CAD build for the part. Positions are in the model's coordinates, mm. Face numbers are marked on the shaded views. A direction names the side the tool comes from. Round coordinates to 2 decimals unless told otherwise and drop trailing zeros. Write each loop counter-clockwise with the first axis right and the second up, starting at its lowest first coordinate (ties: lowest second). Pieces come first, ordered by that corner, then holes. Notation, with made-up numbers: (26.5, 82) -> (67.5, 82) arc R28 ccw to (67.5, 121) -> close; hole circle Ø10 at (51.25, 38.5). An arc over 180 degrees is marked (long way). Put each result on its own line as item: value. Start each with the question number.
1. Saw through at D-D on x = 56.5. List the corners of the cut face in (y, z), and give its area (3 significant figures).
2. Saw through at A-A on y = 4.5. List the corners of the cut face in (x, z).
3. Saw through at B-B on z = 2.25. List the corners of the cut face in (x, y).
4. Saw through at C-C on x = 12.5. List the corners of the cut face in (y, z), and give its area (3 significant figures).
5. Pull direction X, two halves, no side cores. Call the marked faces 3, 4 and 5: pulls with the +X half, pulls with the -X half, needs draft (parallel to the pull), parting line crosses it, or undercut.
6. Flat gauge pins, fed straight in: P1, Ø1.2, axis at x = 2, z = 0.5, coming from the +Y side; P2, Ø3, axis at y = 0.5, z = 2.5, coming from the +X side; P3, Ø4, axis at y = 6, z = -3.5, coming from the +X side; P4, Ø4, axis at y = 6, z = 6, coming from the +X side. Where does each tip first touch, or does it go through?
7. Drill centre lines: line 1 (X direction, y = 0.25, z = 4.75); line 2 (Y direction, x = 49, z = 1.5); line 3 (X direction, y = 2, z = -5.25). Where is each one in solid material? Low to high. Write a range as from..to.
8. 3-axis set-ups, long thin cutter, end or side, ignore diameter. For the marked faces 1 and 2: which of +Z, -Z, +X, -X, +Y, -Y reach the whole face in a straight line?
from build123d import *

# Parameters (mm, degrees)
BOSS_EXTRUDE1_DEPTH = 5.5
SKETCH2_W           = 53.34
SKETCH2_H           = 3
BOSS_EXTRUDE2_DEPTH = 13.95
SCALE1_SCALE        = 0.98


with BuildPart() as part:
    # Sketch1 → Boss-Extrude1 (new, symmetric)
    with BuildSketch(Plane.XY):
        with BuildLine():
            Line((0, 0), (2.5, 0))
            Line((2.5, 0), (2.5, -0.54))
            Line((2.5, -0.54), (55.84, -0.54))
            Line((55.84, -0.54), (55.84, 1.698))
            Line((55.84, 1.698), (57.84, 1.698))
            Line((57.84, 1.698), (58.54, 1.698))
            ThreePointArc((58.54, 1.698), (59.247106781, 1.990893219), (59.54, 2.698))
            Line((59.54, 2.698), (59.54, 7.579046555))
            ThreePointArc((59.54, 7.579046555), (61.34, 9.379046555), (63.14, 7.579046555))
            Line((63.14, 7.579046555), (63.14, -0.54))
            Line((63.14, -0.54), (66.14, -0.54))
            Line((66.14, -0.54), (66.14, 0.46))
            Line((66.14, 0.46), (63.84, 0.46))
            Line((63.84, 0.46), (63.84, 2.16))
            Line((63.84, 2.16), (65.34, 2.16))
            Line((65.34, 2.16), (63.84, 7.758076211))
            Line((63.84, 7.758076211), (63.84, 7.579046555))
            ThreePointArc((63.84, 7.579046555), (61.34, 10.079046555), (58.84, 7.579046555))
            Line((58.84, 7.579046555), (58.84, 2.46))
            Line((58.84, 2.46), (55.84, 2.46))
            Line((55.84, 2.46), (2.5, 2.46))
            Line((2.5, 2.46), (2.5, 0.5))
            Line((2.5, 0.5), (0, 0.5))
            Line((0, 0.5), (0, 0))
        make_face()
    extrude(amount=BOSS_EXTRUDE1_DEPTH, both=True)

    # Sketch2 → Boss-Extrude2 (add, symmetric)
    with BuildSketch(Plane.XY):
        with Locations((29.17, 0.96)):
            Rectangle(SKETCH2_W, SKETCH2_H)
    extrude(amount=BOSS_EXTRUDE2_DEPTH, both=True)


with BuildPart() as part_1:
    # Scale1: scaled about (30.852442752, 1.144909894, 0)
    add(part.part.scale(SCALE1_SCALE).moved(Location((0.617048855, 0.022898198, 0))))


solid = part_1.part
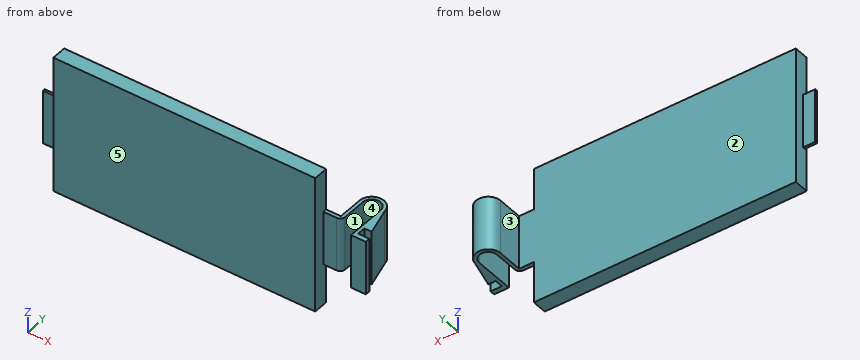
Return value:
1. outline: (1.69, -5.39) -> (2.43, -5.39) -> (2.43, 5.39) -> (1.69, 5.39) -> close
1. area: 8.05 mm^2
2. outline: (58.28, -5.39) -> (58.97, -5.39) -> (58.97, 5.39) -> (58.28, 5.39) -> close; (62.49, -5.39) -> (64.02, -5.39) -> (64.02, 5.39) -> (62.49, 5.39) -> close
3. outline: (0.62, 0.02) -> (3.07, 0.02) -> (3.07, -0.51) -> (55.34, -0.51) -> (55.34, 1.69) -> (57.99, 1.69) arc R0.98 ccw to (58.97, 2.67) -> (58.97, 7.45) arc R1.76 cw to (62.49, 7.45) -> (62.49, -0.51) -> (65.43, -0.51) -> (65.43, 0.47) -> (63.18, 0.47) -> (63.18, 2.14) -> (64.65, 2.14) -> (63.18, 7.63) -> (63.18, 7.45) arc R2.45 ccw to (58.28, 7.45) -> (58.28, 2.43) -> (3.07, 2.43) -> (3.07, 0.51) -> (0.62, 0.51) -> close
4. outline: (-0.51, -13.67) -> (2.43, -13.67) -> (2.43, 13.67) -> (-0.51, 13.67) -> close
4. area: 80.4 mm^2
5. face 3: pulls with the -X half
5. face 4: undercut
5. face 5: needs draft
6. P1: stops at y = 0.51
6. P2: stops at x = 65.43
6. P3: stops at x = 64.15
6. P4: stops at x = 64.13
7. line 1: x = 0.62..55.34, 62.49..65.43
7. line 2: y = -0.51..2.43
7. line 3: x = 3.07..58.7, 62.49..63.18
8. face 1: +Z, -Z, -Y
8. face 2: +Z, -Z, -X, +Y
